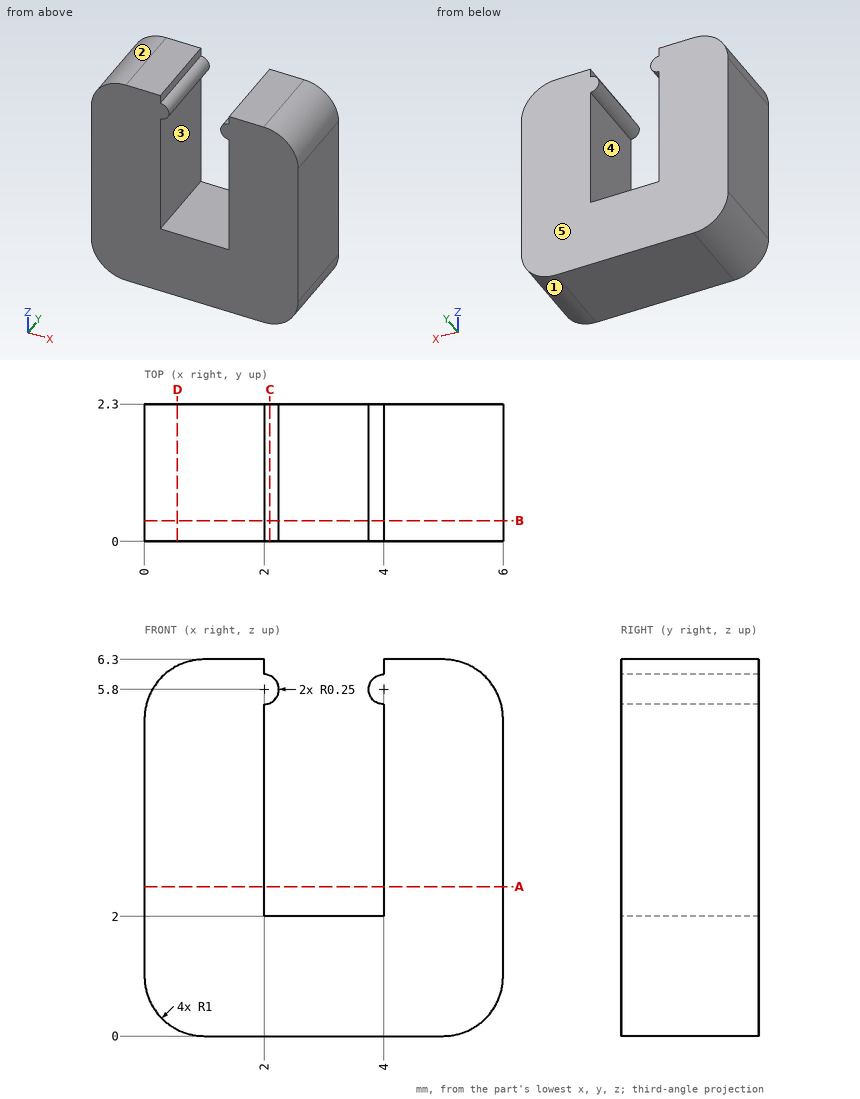
Study the drawing (mm; zero at the part's minimum x, y, z) and answer. A direction names the side the tool comes from. Coordinates: 2 decimals unless noted, no trailing zeros. Order: outer loops, then holes, each group sorted by start corner. A loop starts at its lowest first (then second) coordinate and runs counter-clockwise, first axis right, second up. Notation, with made-up numbers: (54, 37.25) -> (78, 37.25) arc R31 ccw to (78, 74.25) -> close; hole circle Ø9 at (3, 12.5). An arc over 180 degrees is marked (long way). Answer in a Markdown table with one row per item. Add a question column.
Item 1: This flat-tipped pin is pushed along its axis until it touches: P1, Ø1, axis at x = 3, y = 1.5, coming from the +Z side. Where does it stop, or does it pass through?
Item 2: Find the intervals of material crossed by L1, parallel to X at y = 0.35, z = 3.75; L2, parallel to X at y = 2.05, z = 5.75; L3, parallel to Z at x = 3.95, y = 1.4, in increasing order. Write a range as from..to.
Item 3: Find section C-C (x = 2.1). Write down the section's boundary in (y, z).
Item 4: Determine the mould class of the marked faces 1, 2 and 3 for opening direction Z: +Z half, -Z half, draft (parallel to the pull), parting line (faces both ways), or undercut.
Item 5: Find section B-B (y = 0.35). Write down the section's boundary in (x, z).
Item 6: Find section A-A (z = 2.5). Write down the section's boundary in (x, y).
Item 7: Find section D-D (x = 0.55). Write down the section's boundary in (y, z), then the cut area to 3 significant figures.
Item 8: Which of the six approach directions +Z, -Z, +X, -X, +Y, -Y give full straight-line access (tool end or side, diameter ignored) to the marked faces 4 and 5?
Result set:
| question | item | result |
|---|---|---|
| 1 | P1 | stops at z = 2 |
| 2 | L1 | x = 0..2, 4..6 |
| 2 | L2 | x = 0.11..2.24, 3.76..5.89 |
| 2 | L3 | z = 0..2, 5.56..6.04 |
| 3 | outline | (0, 0) -> (2.3, 0) -> (2.3, 2) -> (0, 2) -> close; (0, 5.57) -> (2.3, 5.57) -> (2.3, 6.03) -> (0, 6.03) -> close |
| 4 | face 1 | -Z half |
| 4 | face 2 | +Z half |
| 4 | face 3 | undercut |
| 5 | outline | (0, 1) arc R1 ccw to (1, 0) -> (5, 0) arc R1 ccw to (6, 1) -> (6, 5.3) arc R1 ccw to (5, 6.3) -> (4, 6.3) -> (4, 6.05) arc R0.25 ccw to (4, 5.55) -> (4, 2) -> (2, 2) -> (2, 5.55) arc R0.25 ccw to (2, 6.05) -> (2, 6.3) -> (1, 6.3) arc R1 ccw to (0, 5.3) -> close |
| 6 | outline | (0, 0) -> (2, 0) -> (2, 2.3) -> (0, 2.3) -> close; (4, 0) -> (6, 0) -> (6, 2.3) -> (4, 2.3) -> close |
| 7 | outline | (0, 0.11) -> (2.3, 0.11) -> (2.3, 6.19) -> (0, 6.19) -> close |
| 7 | area | 14.0 mm² |
| 8 | face 4 | +Y, -Y |
| 8 | face 5 | +Z, -Z, +X, -X, +Y |
